The model under review builds one solid part; all positions refer to its coordinate system, in mm. A direction names the side the tool comes from. Give positions to 0.01 mm unless a question says otherwise; leave off trailing zeros. Order: outer loops, then holes, each group sorted by start corner. A loop starts at its lowest first (then second) coordinate and runs counter-clockwise, first axis right, second up.
```python
from build123d import *

# Parameters (mm, degrees)
SKETCH1_R           = 7.575
SKETCH1_R_2         = 4.575
BOSS_EXTRUDE1_DEPTH = 12
BOSS_EXTRUDE2_START = 2
SKETCH2_R           = 7.575
BOSS_EXTRUDE2_DEPTH = 2
SKETCH4_W           = 8
SKETCH4_H           = 8
BOSS_EXTRUDE3_DEPTH = 2.25
SKETCH5_R           = 1.5
CUT_EXTRUDE1_DEPTH  = 18.260105735
FILLET1_R           = 3.5
FILLET2_R           = 1.5
FILLET3_R           = 0.8
CHAMFER1_SIZE2      = 2
CHAMFER1_SIZE       = 1.154700538


with BuildPart() as part:
    # Sketch1 → Boss-Extrude1 (new body)
    with BuildSketch(Plane.XY):
        Circle(SKETCH1_R)
        Circle(SKETCH1_R_2, mode=Mode.SUBTRACT)
    extrude(amount=BOSS_EXTRUDE1_DEPTH)

    # Sketch2 → Boss-Extrude2 (add)
    with BuildSketch(Plane(origin=(0, 0, 0), x_dir=(-1, 0, 0), z_dir=(0, 0, -1)).offset(BOSS_EXTRUDE2_START)):
        Circle(SKETCH2_R)
    extrude(amount=-BOSS_EXTRUDE2_DEPTH)

    # Sketch4 → Boss-Extrude3 (add, symmetric)
    with BuildSketch(Plane(origin=(0, 0, 0), x_dir=(0, 0, -1), z_dir=(1, 0, 0))):
        with Locations((6, 0)):
            Rectangle(SKETCH4_W, SKETCH4_H)
    extrude(amount=BOSS_EXTRUDE3_DEPTH, both=True)

    # Sketch5 → Cut-Extrude1 (cut, through all)
    with BuildSketch(Plane(origin=(2.25, 0, 0), x_dir=(0, 0, -1), z_dir=(1, 0, 0))):
        with Locations((6.5, 0)):
            Circle(SKETCH5_R)
    extrude(amount=-CUT_EXTRUDE1_DEPTH, mode=Mode.SUBTRACT)

    # Fillet1
    fillet1_edges = [part.edges().sort_by_distance(p)[0] for p in [
        (0, -4, -10),
        (0, 4, -10),
    ]]
    fillet(fillet1_edges, radius=FILLET1_R)

    # Fillet2
    fillet2_edges = [part.edges().sort_by_distance(p)[0] for p in [
        (0, 4, -2),
        (0, -4, -2),
    ]]
    fillet(fillet2_edges, radius=FILLET2_R)

    # Fillet3
    fillet3_edges = [part.edges().sort_by_distance(p)[0] for p in [
        (-2.25, 0, -2),
        (2.25, 0, -2),
    ]]
    fillet(fillet3_edges, radius=FILLET3_R)

    # Chamfer1
    chamfer1_edges = [part.edges().sort_by_distance(p)[0] for p in [
        (7.575, 0, -2),
    ]]
    chamfer1_side = [part.faces().sort_by_distance(p)[0] for p in [
        (7.551905989, 0, -2),
    ]]
    chamfer(chamfer1_edges, length=CHAMFER1_SIZE - 0.0001, length2=CHAMFER1_SIZE2 - 0.0001, reference=chamfer1_side[0])  # a hair under: the kernel refuses the full size


solid = part.part
```
Item 1: Take a section at D-D (z = -3.25). Give the boundary of the cut face in (x, y).
Values found:
outline: (-2.25, -4.02) - (2.25, -4.02) - (2.25, 4.02) - (-2.25, 4.02) - close
Item 2: For faces 4 (the flat face through (-2.25, 0.1, -4.7)), 5 (the flat face through (2.25, 0.1, -4.7)), 6 (the flat face through (0, 0, 0)), 7 (the flat face through (0, 4, -5)), 8 (the flat face through (5, 0, 12)), list the 3-axis set-ups (+Z, -Z, +X, -X, +Y, -Y) from which the entire face can be reached by the end or side of a thin tool; tool diameter is ignored.
Values found:
face 4: -Z, -X, +Y, -Y
face 5: -Z, +X, +Y, -Y
face 6: +Z
face 7: -Z, +X, -X, +Y
face 8: +Z, +X, -X, +Y, -Y
Item 3: Take a section at A-A (y = 0). Give the boundary of the cut face in (x, z) (3 decimals).
Values found:
outline: (-7.575, 0) - (-6.42, -2) - (-3.05, -2) arc R0.8 cw to (-2.25, -2.8) - (-2.25, -5) - (2.25, -5) - (2.25, -2.8) arc R0.8 cw to (3.05, -2) - (6.42, -2) - (7.575, 0) - (7.575, 12) - (4.575, 12) - (4.575, 0) - (-4.575, 0) - (-4.575, 12) - (-7.575, 12) - close; (-2.25, -10) - (2.25, -10) - (2.25, -8) - (-2.25, -8) - close
Item 4: For line 1 (Y direction, x = 0, z = 6) (3 decimals); line 2 (X direction, y = -4, z = 0.5); line 3 (Y direction, x = 0.9, z = -6.5), list the stretches that pass through material, from the lowest coordinate up.
Values found:
line 1: y = -7.575 to -4.575, 4.575 to 7.575
line 2: x = -6.43 to -2.22, 2.22 to 6.43
line 3: y = -4 to -1.5, 1.5 to 4
Item 5: Take a section at B-B (x = 0). Give the boundary of the cut face in (y, z) (3 decimals), and give its area (3 significant figures).
Values found:
outline: (-7.575, 0) - (-6.42, -2) - (-5.5, -2) arc R1.5 cw to (-4, -3.5) - (-4, -6.5) arc R3.5 ccw to (-0.5, -10) - (0.5, -10) arc R3.5 ccw to (4, -6.5) - (4, -3.5) arc R1.5 cw to (5.5, -2) - (6.42, -2) - (7.575, 0) - (7.575, 12) - (4.575, 12) - (4.575, 0) - (-4.575, 0) - (-4.575, 12) - (-7.575, 12) - close; hole circle Ø3 at (0, -6.5)
area: 153 mm2
Item 6: Clearance check with flat-ended pins moving along their axes: pin 1 Ø4 at (y, z) = (3.5, 7) entering from -X (3 decimals); pin 2 Ø8 at (y, z) = (-1, -7) entering from +X; pin 3 Ø6 at (x, z) = (4.5, -1.5) entering from +Y. State where each tip first meets the part, or that it passes through.
Values found:
pin 1: stops at x = -7.425
pin 2: stops at x = 2.25
pin 3: stops at y = 7.33
Item 7: Take a section at C-C (z = 4.5). Give the boundary of the cut face in (x, y) (3 decimals).
Values found:
outline: circle Ø15.15 at (0, 0); hole circle Ø9.15 at (0, 0)
Item 8: Draft analysis for pull direction Z (two halves, no side actions). For faces 1 (the cylindrical face through (-0.04, 4.45, -2.43)), 2 (the flat face through (0, -4, -5)), 3 (the cylindrical face through (0, 0, -5)), state which applies: released by +Z, released by -Z, zero draft, split by the parting line, or undercut.
Values found:
face 1: released by -Z
face 2: zero draft
face 3: undercut
